CAD build for the part. Positions are in the model's coordinates, mm. Face numbers are marked on the shaded views. A direction names the side the tool comes from. Coordinates: 2 decimals unless noted, no trailing zeros. Loops run counter-clockwise (first coordinate to the right, second up) from the corner with the lowest first, then second, coordinate; pieces in that order, holes last.
1) Saw through at D-D, the plane x = 17. Write the cut outline in (y, z), and give its area (3 significant figures).
2) Wall check: line 1 along Y through (x, z) = (52, 1.45); line 2 along Y through (x, z) = (70.6, 25); line 3 along X through (y, z) = (9, 20). Give the ranges that are in metal, low to high.
3) Saw through at A-A, the plane z = 18. Write the cut outline in (x, y), and give its area (3 significant figures).
4) Which spindle directions (+Z, -Z, +X, -X, +Y, -Y) get a long thin tool onto all of the face, cutting with end or side? Do the marked faces 1 and 2. Say none if no direction does.
5) Saw through at B-B, the plane y = 42. Write the cut outline in (x, z), and give its area (3 significant figures).
6) Saw through at C-C, the plane z = 25. Give the number of separate pieces and of enclosed holes in the cut face, and give its area (3 significant figures).
7) Pin check, flat tips, straight feed: pin 1 Ø8 at (x, y) = (18, 66) entering from +Z; pin 2 Ø1 at (x, z) = (35, 1) entering from +Y; pin 3 Ø6 at (y, z) = (110, 25) entering from -X. Stop position of each tip, or through.
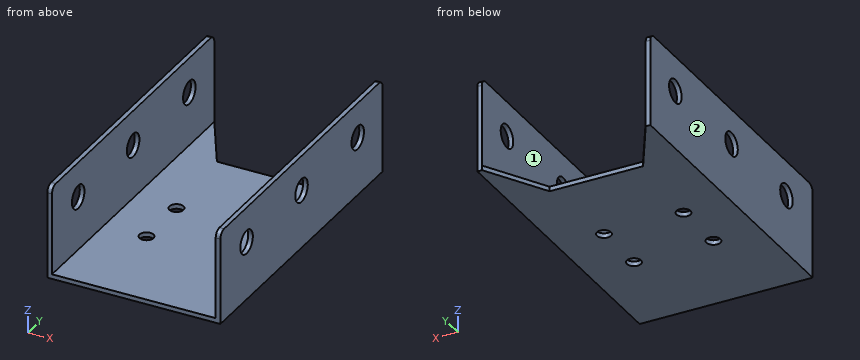
```python
from build123d import *

# Parameters (mm, degrees)
CYLINDER001_R     = 5
CYLINDER001_DEPTH = 100
CYLINDER002_R     = 5
CYLINDER002_DEPTH = 100
CYLINDER_R        = 5
CYLINDER_DEPTH    = 100
BOX001_W          = 2
BOX001_H          = 130
BOX001_DEPTH      = 40
BOX_W             = 2
BOX_H             = 130
BOX_DEPTH         = 40
SKETCH_R          = 3
EXTRUDE_DEPTH     = 2
FILLET_R          = 3


with BuildPart() as obj1:
    # Cylinder001 → Cylinder001 (new body)
    with BuildSketch(Plane(origin=(-10, 65, 25), x_dir=(0, 0, -1), z_dir=(1, 0, 0))):
        Circle(CYLINDER001_R)
    extrude(amount=CYLINDER001_DEPTH)


with BuildPart() as obj2:
    # Cylinder002 → Cylinder002 (new body)
    with BuildSketch(Plane(origin=(-10, 21, 25), x_dir=(0, 0, -1), z_dir=(1, 0, 0))):
        Circle(CYLINDER002_R)
    extrude(amount=CYLINDER002_DEPTH)


with BuildPart() as fusion001:
    # Cylinder → Cylinder (new body)
    with BuildSketch(Plane(origin=(-10, 110, 25), x_dir=(0, 0, -1), z_dir=(1, 0, 0))):
        Circle(CYLINDER_R)
    extrude(amount=CYLINDER_DEPTH)

    # Fusion001: union obj1, obj2
    add(obj1.part)
    add(obj2.part)


with BuildPart() as krychle001:
    # Box001 → Box001 (new body)
    with BuildSketch(Plane(origin=(70, 0, 0), x_dir=(1, 0, 0), z_dir=(0, 0, 1))):
        with Locations((1, 65)):
            Rectangle(BOX001_W, BOX001_H)
    extrude(amount=BOX001_DEPTH)


with BuildPart() as cut:
    # Box → Box (new body)
    with BuildSketch(Plane(origin=(-2, 0, 0), x_dir=(1, 0, 0), z_dir=(0, 0, 1))):
        with Locations((1, 65)):
            Rectangle(BOX_W, BOX_H)
    extrude(amount=BOX_DEPTH)

    # Fusion: union Krychle001
    add(krychle001.part)

    # Cut: cut Fusion001
    add(fusion001.part, mode=Mode.SUBTRACT)


with BuildPart() as fillet_body:
    # Sketch → Extrude (new body)
    with BuildSketch(Plane.XY):
        Polygon((0, 130), (0, 0), (70, 0), (70, 130), (55, 104), (15, 104), align=None)
        with Locations((52, 66)):
            Circle(SKETCH_R, mode=Mode.SUBTRACT)
        with Locations((18, 42)):
            Circle(SKETCH_R, mode=Mode.SUBTRACT)
        with Locations((52, 42)):
            Circle(SKETCH_R, mode=Mode.SUBTRACT)
        with Locations((18, 66)):
            Circle(SKETCH_R, mode=Mode.SUBTRACT)
    extrude(amount=EXTRUDE_DEPTH)

    # Fusion002: union Cut
    add(cut.part)

    # Fillet
    fillet_edges = [fillet_body.edges().sort_by_distance(p)[0] for p in [
        (71, 130, 40),
        (71, 0, 40),
        (-1, 130, 40),
        (-1, 0, 40),
    ]]
    fillet(fillet_edges, radius=FILLET_R)


solid = fillet_body.part
```
Data:
1. outline: (0, 0) - (39.17, 0) - (39.17, 2) - (0, 2) - close; (44.83, 0) - (63.17, 0) - (63.17, 2) - (44.83, 2) - close; (68.83, 0) - (104, 0) - (104, 2) - (68.83, 2) - close
1. area: 185 mm2
2. line 1: y = 0 to 39, 45 to 63, 69 to 104
2. line 2: y = 0 to 16, 26 to 60, 70 to 105, 115 to 130
2. line 3: x = -2 to 0, 70 to 72
3. outline: (-2, 0) - (0, 0) - (0, 130) - (-2, 130) - close; (70, 0) - (72, 0) - (72, 130) - (70, 130) - close
3. area: 520 mm2
4. face 1: +Z, +Y, -Y
4. face 2: +Z, -Z, -X, +Y, -Y
5. outline: (-2, 0) - (15, 0) - (15, 2) - (0, 2) - (0, 40) - (-2, 40) - close; (21, 0) - (49, 0) - (49, 2) - (21, 2) - close; (55, 0) - (72, 0) - (72, 40) - (70, 40) - (70, 2) - (55, 2) - close
5. area: 276 mm2
6. separate pieces: 8
6. enclosed holes: 0
6. area: 400 mm2
7. pin 1: stops at z = 2
7. pin 2: stops at y = 104
7. pin 3: passes through
